The listing builds one solid part. Answer for the finished solid, in the listing's coordinates (mm). Face numbers are marked on the shaded views. A direction names the side the tool comes from. Coordinates: 2 decimals unless noted, no trailing zeros. Write each loop counter-clockwise with the first axis right and the second up, starting at its lowest first coordinate (ties: lowest second). Pieces come first, ordered by that corner, then holes.
(1) Given P1, Ø1, axis at x = 14.5, z = -17, coming from the -Y side; P2, Ø2, axis at x = 17, y = 17.5, coming from the +Z side; P3, Ø10, axis at x = 2.5, z = 4.5, coming from the -Y side; P4, Ø1, axis at x = 9, z = -3.5, coming from the +Y side, each flat-ended and moving along its own axis, determine where each tip first touches the part or whether it passes through.
(2) Straight lines are drawn through the part: line 1 (Z direction, x = 17.25, y = 1); line 2 (Y direction, x = 2.1, z = 0); line 3 (Z direction, x = 18.1, y = 0). For each, find the intervals that lie inside material, in ascending order.
(3) Which of the six approach directions +Z, -Z, +X, -X, +Y, -Y give full straight-line access (tool end or side, diameter ignored) to the marked faces 1 and 2?
(4) The part is cut by section A-A on y = 0. Determine the outline of the cut face in (x, z), plus the area to 3 significant figures.
(5) The part is cut by section B-B on x = 1.5. Determine the outline of the cut face in (y, z), plus the area to 3 significant figures.
(6) The part is cut by section D-D on x = 12.5. Determine the outline of the cut face in (y, z), plus the area to 3 significant figures.
(7) The part is cut by section C-C on x = 6.75. Determine the outline of the cut face in (y, z).
(8) For a pull along Y with two mould halves and no side action, classify the marked faces 3, 4 and 5 as +Y half, -Y half, draft (parallel to the pull), parting line (faces both ways), or undercut.
Autodesk Inventor part; units mm, degrees
ref_plane "YZ Plane" through (0, 0, 0) normal (1, 0, 0) x (0, 1, 0)
ref_plane "XZ Plane" through (0, 0, 0) normal (0, 1, 0) x (-1, 0, 0)
ref_plane "XY Plane" through (0, 0, 0) normal (0, 0, 1) x (1, 0, 0)
sketch "Эскиз5" plane through (0, 0, 0) normal (0, 0, 1) x (1, 0, 0)
  line L0 (0, 0) -> (20, 0)
  line L1 (20, 0) -> (20, 25)
  line L2 (16, 29) -> (4, 29)
  line L3 (0, 25) -> (0, 0)
  line L4 (4, 29) -> (0, 25)
  line L5 (16, 29) -> (20, 25)
  point P0 (20, 29)
  point P1 (0, 29)
  dimension "d23" = 20
  dimension "d24" = 29
  dimension "d25" = 4
  dimension "d26" = 4
  dimension "d27" = 4
  dimension "d28" = 4
revolve "Вращение3" add sketch "Эскиз5" angle 360 about axis through (0, 0, 0) along (1, 0, 0)
sketch "Эскиз6" plane through (0, 0, 0) normal (0, 0, 1) x (1, 0, 0)
  line L0 (0, -25) -> (0, 25) construction
  line L1 (0, 4) -> (9, 4)
  line L2 (9, 4) -> (9, -4)
  line L3 (9, -4) -> (0, -4)
  line L4 (0, -4) -> (0, 4)
  point P0 (0, 0)
  point P1 (0, 0)
  point P2 (0, 0)
  dimension "d30" = 9
  dimension "d31" = 8
extrude "Выдавливание2" cut sketch "Эскиз6" along normal through all both and the other way through all
sketch "Эскиз7" plane through (0, 0, 0) normal (-1, 0, 0) x (0, 0, 1)
  line L0 (0, 0) -> (0, 20) construction
  dimension "d34" = 20
hole "Отверстие2" at (0, 20, 0) direction (1, 0, 0) diameter 4 depth 4 tip angle 118
sketch "Эскиз8" plane through (0, 0, 0) normal (0, 0, 1) x (1, 0, 0)
  line L0 (20, -25) -> (20, 25) construction
  line L1 (20, 25) -> (16, 25)
  line L2 (16, 25) -> (16, 21.5)
  line L3 (16, 21.5) -> (20, 21.5)
  line L4 (20, 21.5) -> (20, 25)
  line L5 (0, 0) -> (20, 0)
  dimension "d42" = 4
  dimension "d43" = 3.5
revolve "Вращение4" cut sketch "Эскиз8" angle 360 about axis through (0, 0, 0) along (1, 0, 0)
properties part number "711118"
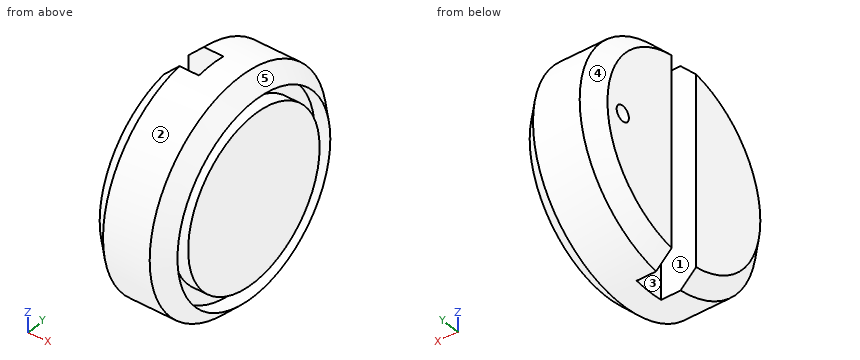
Model answer:
1. P1: stops at y = -23.85
1. P2: stops at z = 23.33
1. P3: stops at y = -29
1. P4: stops at y = 28.84
2. line 1: z = -27.73 to -24.98, -21.48 to 21.48, 24.98 to 27.73
2. line 2: y = -27.1 to -4, 4 to 18, 22 to 27.1
2. line 3: z = -26.9 to -25, -21.5 to 21.5, 25 to 26.9
3. face 1: +Z, -Z, -X
3. face 2: +X, -X
4. outline: (9, -29) - (16, -29) - (20, -25) - (16, -25) - (16, -21.5) - (20, -21.5) - (20, 21.5) - (16, 21.5) - (16, 25) - (20, 25) - (16, 29) - (9, 29) - close
4. area: 594 mm2
5. outline: (-4, -26.2) - (-4, 26.2) arc R26.5 ccw to start; (4, -26.2) arc R26.5 ccw to (4, 26.2) - close; hole circle Ø4 at (20, 0)
5. area: 1,770 mm2
6. outline: circle Ø58 at (0, 0)
6. area: 2,640 mm2
7. outline: (-4, -28.72) - (-4, 28.72) arc R29 ccw to start; (4, -28.72) arc R29 ccw to (4, 28.72) - close
8. face 3: undercut
8. face 4: +Y half
8. face 5: parting line
